Can you work these out from the model? Positions are in its coordinate system, mm. Face numbers are marked on the shaded views. A direction names the side the tool comes from. Round coordinates to 2 decimals unless told otherwise and drop trailing zeros. Write each loop counter-clockwise with the first axis right and the second up, starting at its lowest first coordinate (ties: lowest second). Pieces come first, ordered by that corner, then holes. Notation, with made-up numbers: (31, 3.25) -> (76, 3.25) arc R31 cw to (76, 31.25) -> close; hole circle Ø9 at (53, 9). An arc over 180 degrees is marked (long way). Use CSV: the item, a comma, the result in double quotes.
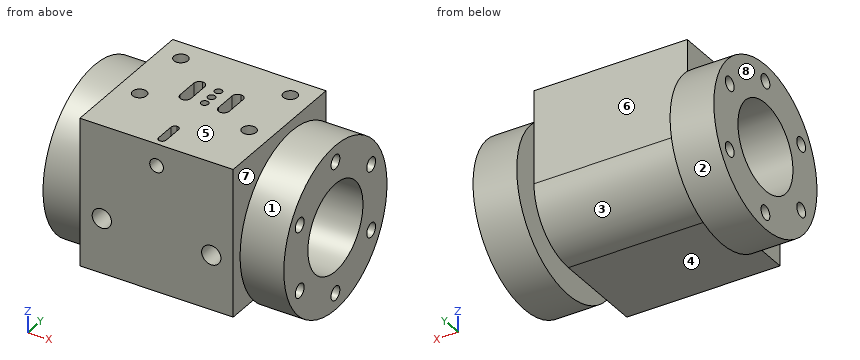
```python
from build123d import *

# Parameters (mm, degrees)
F0_W             = 34.925
F0_H             = 25.4
F1_DEPTH         = 25.4
F3_DEPTH         = 6.35
F5_DEPTH         = 6.35
F6_D             = 12.7
F9_DEPTH         = 22.225
F11_D            = 2.794
F11_DEPTH        = 4.7625
F11_TIP          = 0.8394022848
F13_D            = 2.032
F13_DEPTH        = 4.7625
F13_TIP          = 0.6104743889
F16_D            = 2.032
F16_DEPTH        = 4.7625
F16_TIP          = 0.6104743889
F16_ON_F15_D     = 2.032
F16_ON_F15_DEPTH = 4.7625
F16_ON_F15_TIP   = 0.6104743889
F17_W            = 1.5875
F17_H            = 4.7625
F18_DEPTH        = 3.175
F19_R            = 0.79374
F20_R            = 0.9921875
F21_DEPTH        = 15.52488
F22_R            = 0.5461
F22_W            = 1.0922
F22_H            = 3.96875
F23_DEPTH        = 3.175
F24_R            = 0.54609


# Not quite as in the source:
# - a fillet or chamfer is up to 0.001 mm smaller than in the source, because OpenCascade refuses the exact size


with BuildPart() as f1:
    # F0 (on Top) → F1 (new body)
    with BuildSketch(Plane.XY):
        Rectangle(F0_W, F0_H)
    extrude(amount=F1_DEPTH)

    # F2 (on face) → F3 (cut)
    with BuildSketch(Plane.YZ.offset(17.4625)):
        with BuildLine():
            Line((-12.7, 25.4), (-12.7, 0))
            Line((-12.7, 0), (0.79375, 0))
            ThreePointArc((0.79375, 0), (-7.6252401135, 20.3252401135), (12.7, 11.90625))
            Line((12.7, 11.90625), (12.7, 25.4))
            Line((12.7, 25.4), (-12.7, 25.4))
        make_face()
        with BuildLine():
            ThreePointArc((12.7, 11.90625), (9.2127401135, 3.4872598865), (0.79375, 0))
            Line((0.79375, 0), (12.7, 0))
            Line((12.7, 0), (12.7, 11.90625))
        make_face()
    extrude(amount=-F3_DEPTH, mode=Mode.SUBTRACT)

    # F4 (on face) → F5 (cut)
    with BuildSketch(Plane(origin=(-17.4625, 0, 0), x_dir=(0, -1, 0), z_dir=(-1, 0, 0))):
        with BuildLine():
            ThreePointArc((11.1125, 11.90625), (7.6252401135, 3.4872598865), (-0.79375, 0))
            Line((-0.79375, 0), (12.7, 0))
            Line((12.7, 0), (12.7, 25.4))
            Line((12.7, 25.4), (-12.7, 25.4))
            Line((-12.7, 25.4), (-12.7, 11.9062500146))
            ThreePointArc((-12.7, 11.9062500146), (-0.7937499927, 23.8125), (11.1125, 11.90625))
        make_face()
        with BuildLine():
            Line((-12.7, 11.9062500146), (-12.7, 0))
            Line((-12.7, 0), (-0.79375, 0))
            ThreePointArc((-0.79375, 0), (-9.2127401186, 3.4872598916), (-12.7, 11.9062500146))
        make_face()
    extrude(amount=-F5_DEPTH, mode=Mode.SUBTRACT)

    # F6 (through all)
    with Locations(Plane.YZ.offset(17.4625)):
        with Locations((0.79375, 11.90625)):
            Hole(F6_D / 2)

    # F8 (on offset) → F9 (cut)
    with BuildSketch(Plane.YZ.offset(11.1125)):
        with BuildLine():
            Line((-12.7, 3.96875), (-12.7, 0))
            Line((-12.7, 0), (12.7, 0))
            Line((12.7, 0), (12.7, 25.4))
            Line((12.7, 25.4), (8.73125, 25.4))
            Line((8.73125, 25.4), (8.73125, 11.90625))
            ThreePointArc((8.73125, 11.90625), (6.4064100757, 6.2935899243), (0.79375, 3.96875))
            Line((0.79375, 3.96875), (-12.7, 3.96875))
        make_face()
    extrude(amount=-F9_DEPTH, mode=Mode.SUBTRACT)

    # F11
    with Locations(Plane.XZ.offset(12.7)):
        with Locations((-7.9375, 11.90625), (7.9375, 11.90625)):
            Hole(F11_D / 2, depth=F11_DEPTH)
            with Locations((0, 0, -(F11_DEPTH + F11_TIP / 2))):  # 118° drill point
                Cone(0, F11_D / 2, F11_TIP, mode=Mode.SUBTRACT)

    # F13
    with Locations(Plane.XY.offset(25.4)):
        with Locations((-7.9375, 5.55625), (7.9375, 5.55625), (7.9375, -3.96875), (-7.9375, -3.96875)):
            Hole(F13_D / 2, depth=F13_DEPTH)
            with Locations((0, 0, -(F13_DEPTH + F13_TIP / 2))):  # 118° drill point
                Cone(0, F13_D / 2, F13_TIP, mode=Mode.SUBTRACT)

    # F16
    with Locations(Plane.YZ.offset(17.4625)):
        with Locations((0.79375, 21.43125), (9.0426419749, 16.6687499934), (9.0426419634, 7.1437499867), (0.793749977, 2.38125), (-7.4551419864, 7.1437500265), (-7.4551419519, 16.6687500331)):
            Hole(F16_D / 2, depth=F16_DEPTH)
            with Locations((0, 0, -(F16_DEPTH + F16_TIP / 2))):  # 118° drill point
                Cone(0, F16_D / 2, F16_TIP, mode=Mode.SUBTRACT)

    # F16 on F15
    with Locations(Plane(origin=(-17.4625, 0, 0), x_dir=(0, -1, 0), z_dir=(-1, 0, 0))):
        with Locations((-0.79375, 21.43125), (-9.042641971, 16.66875), (-9.042641971, 7.14375), (-0.79375, 2.38125), (7.455141971, 7.14375), (7.455141971, 16.66875)):
            Hole(F16_ON_F15_D / 2, depth=F16_ON_F15_DEPTH)
            with Locations((0, 0, -(F16_ON_F15_DEPTH + F16_ON_F15_TIP / 2))):  # 118° drill point
                Cone(0, F16_ON_F15_D / 2, F16_ON_F15_TIP, mode=Mode.SUBTRACT)

    # F17 (on face) → F18 (cut)
    with BuildSketch(Plane.XY.offset(25.4)):
        with Locations((2.778125, 0)):
            Rectangle(F17_W, F17_H)
        with Locations((-2.778125, 0)):
            Rectangle(F17_W, F17_H)
    extrude(amount=-F18_DEPTH, mode=Mode.SUBTRACT)

    # F19 (radius 0.79375 in the source; OpenCascade refuses exactly that, so slightly less here)
    f19_edges = [f1.edges().sort_by_distance(p)[0] for p in [
        (-3.571875, 2.38125, 23.8125),
        (-1.984375, 2.38125, 23.8125),
        (-1.984375, -2.38125, 23.8125),
        (-3.571875, -2.38125, 23.8125),
        (1.984375, -2.38125, 23.8125),
        (3.571875, 2.38125, 23.8125),
        (1.984375, 2.38125, 23.8125),
        (3.571875, -2.38125, 23.8125),
    ]]
    fillet(f19_edges, radius=F19_R)

    # F20 (on face) → F21 (cut)
    with BuildSketch(Plane.XZ.offset(12.7)):
        with Locations((0, 22.225)):
            Circle(F20_R)
    extrude(amount=-F21_DEPTH, mode=Mode.SUBTRACT)

    # F22 (on face) → F23 (cut)
    with BuildSketch(Plane.XY.offset(25.4)):
        Circle(F22_R)
        with Locations((0, 1.5875)):
            Circle(F22_R)
        with Locations((0, -1.5875)):
            Circle(F22_R)
        with Locations((0, -9.921875)):
            Rectangle(F22_W, F22_H)
    extrude(amount=-F23_DEPTH, mode=Mode.SUBTRACT)

    # F24 (radius 0.5461 in the source; OpenCascade refuses exactly that, so slightly less here)
    f24_edges = [f1.edges().sort_by_distance(p)[0] for p in [
        (-0.5461, -7.9375, 24.226689),
        (0.5461, -7.9375, 24.226689),
        (0.5461, -11.90625, 24.226689),
        (-0.5461, -11.90625, 24.226689),
    ]]
    fillet(f24_edges, radius=F24_R)


solid = f1.part
```
Q1. Please list where these lines run through material, in increasing order: probe 1 along Y at (x, z) = (-8, 21); probe 2 along X at (y, z) = (-9.25, 11.75); probe 3 along X at (y, z) = (0, 24.85).
Resolved:
probe 1,"y = -12.7 to -4.98, -2.95 to 4.54, 6.57 to 8.73"
probe 2,"x = -17.46 to -9.33, -6.55 to 6.55, 9.33 to 17.46"
probe 3,"x = -11.11 to -3.57, -1.98 to -0.55, 0.55 to 1.98, 3.57 to 11.11"
Q2. Will these pins go through, and if not, where does the flat tip stop? P1, Ø1.2, axis at x = -7.94, y = -3.97, coming from the +Z side; P2, Ø1.7, axis at x = 7.94, z = 11.91, coming from the +Y side; P3, Ø2, axis at x = -12.5, y = -10, coming from the -Z side.
Resolved:
P1,"stops at z = 20.39"
P2,"stops at y = 8.73"
P3,"stops at z = 5.14"
Q3. Suppose I cut it at A-A (z = 8.75). Write out the boundary of the cut face in (x, y), and give its area (3 significant figures).
Resolved:
outline,"(-17.46, -10.69) -> (-11.11, -10.69) -> (-11.11, -12.7) -> (11.11, -12.7) -> (11.11, -10.69) -> (17.46, -10.69) -> (17.46, -4.72) -> (-17.46, -4.72) -> close; (-17.46, 6.3) -> (17.46, 6.3) -> (17.46, 12.27) -> (11.11, 12.27) -> (11.11, 8.08) -> (-11.11, 8.08) -> (-11.11, 12.27) -> (-17.46, 12.27) -> close"
area,"368 mm^2"
Q4. Suppose I cut it at C-C (z = 19.5). Write out the boundary of the cut face in (x, y), and give its area (3 significant figures).
Resolved:
outline,"(-17.46, -8.38) -> (-11.11, -8.38) -> (-11.11, -12.7) -> (11.11, -12.7) -> (11.11, -8.38) -> (17.46, -8.38) -> (17.46, 9.96) -> (11.11, 9.96) -> (11.11, 8.73) -> (-11.11, 8.73) -> (-11.11, 9.96) -> (-17.46, 9.96) -> close"
area,"709 mm^2"
Q5. If we mould it in two halves opening along X, with no side actions, what happens to the marked faces 6, 7 and 8? For each: released by +X, released by -X, zero draft, split by the parting line, or undercut.
Resolved:
face 6,"undercut"
face 7,"released by +X"
face 8,"released by -X"
Q6. On a 3-axis mill with a long thin cutter (end or side, diameter ignored), from which of +Z, -Z, +X, -X, +Y, -Y can I reach the whole of each face in a straight line? I mean the marked faces 1, 2, 3, 4 and 5. Say none if no direction works.
Resolved:
face 1,"+X"
face 2,"-X"
face 3,"-Z, +Y"
face 4,"-Z, +Y, -Y"
face 5,"+Z, +X, -X, +Y, -Y"
Q7. Suppose I cut it at B-B (x = 15). Write out the boundary of the cut face in (y, z), and give its area (3 significant figures).
Resolved:
outline,"circle Ø23.81 at (0.79, 11.91); hole circle Ø2.03 at (-7.46, 7.14); hole circle Ø2.03 at (-7.46, 16.67); hole circle Ø12.7 at (0.79, 11.91); hole circle Ø2.03 at (0.79, 2.38); hole circle Ø2.03 at (0.79, 21.43); hole circle Ø2.03 at (9.04, 7.14); hole circle Ø2.03 at (9.04, 16.67)"
area,"299 mm^2"
